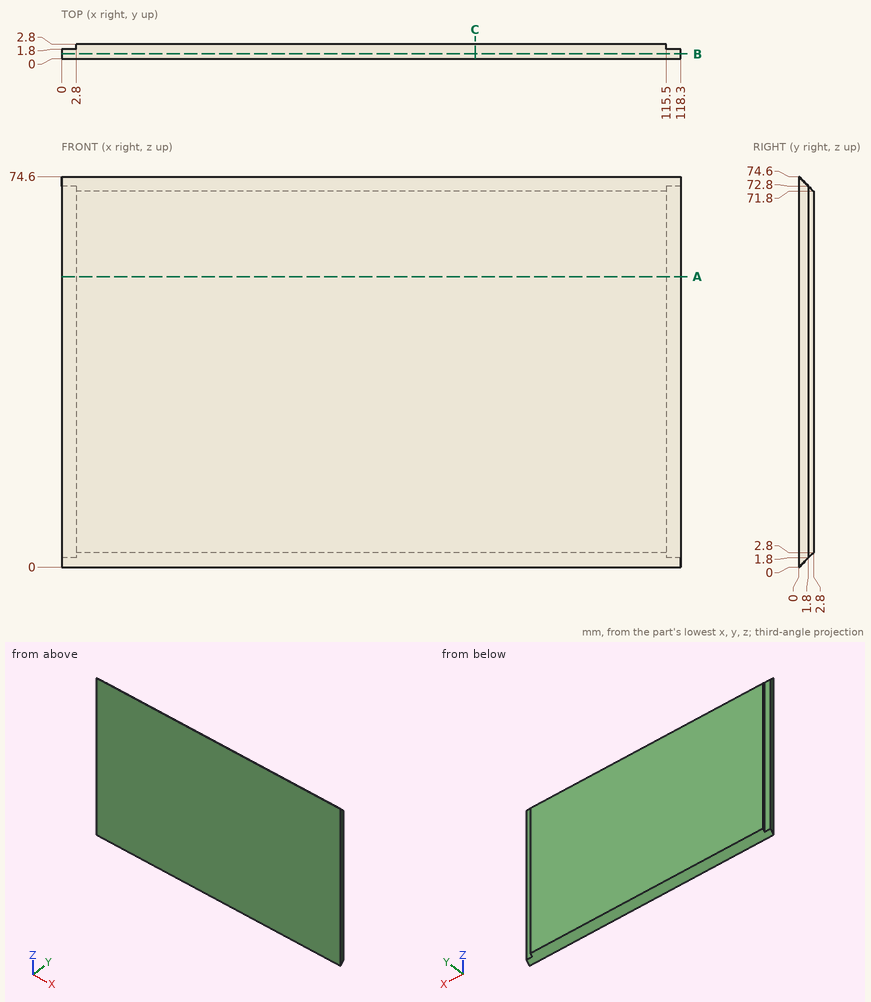
Here's the drawing with two shaded views (mm, measured from the low corner). I have some questions. Round coordinates to 2 decimals unless told otherwise and drop trailing zeros. Write each loop counter-clockwise with the first axis right and the second up, starting at its lowest first coordinate (ties: lowest second). Pieces come first, ordered by that corner, then holes. Notation, with made-up numbers: M -25.5,38.25 L -9.5,38.25 A14 cw -9.5,51.25 Z; hole C 84.25,17 d7. An arc over 180 degrees is marked long. Answer in a Markdown table with one row per item. Add a question column.
Q1. Imagine slicing it at A-A (z = 55.5). Please give me the cut outline in (x, y), then the cut area to 3 significant figures.
Q2. Will these pins go through, and if not, where does the flat tip stop? pin 1 Ø3 at (x, z) = (1, 46.5) entering from +Y; pin 2 Ø1.5 at (x, y) = (56, 1) entering from -Z; pin 3 Ø1.5 at (x, y) = (59.5, 2.5) entering from +Z.
Q3. If I drill on line 1 (X direction, y = 2.2, z = 37); line 2 (Z direction, x = 95.5, y = 0.5); line 3 (Z direction, x = 39.5, y = 1.8), over which ranges is the centre line in solid material (lowest first)? Write a range as from..to.
Q4. Imagine slicing it at B-B (y = 0.9). Please give me the cut outline in (x, z), then the cut area to 3 significant figures.
Q5. Imagine slicing it at C-C (x = 79). Please give me the cut outline in (y, z).
Values:
| question | item | result |
|---|---|---|
| 1 | outline | M 0,0 L 118.3,0 L 118.3,1.8 L 115.5,1.8 L 115.5,2.8 L 2.8,2.8 L 2.8,1.8 L 0,1.8 Z |
| 1 | area | 326 mm^2 |
| 2 | pin 1 | y = 1.8 |
| 2 | pin 2 | z = 0.25 |
| 2 | pin 3 | z = 72.85 |
| 3 | line 1 | 2.8..115.5 |
| 3 | line 2 | 0.5..74.1 |
| 3 | line 3 | 1.8..72.8 |
| 4 | outline | M 0,0.9 L 118.3,0.9 L 118.3,73.7 L 0,73.7 Z |
| 4 | area | 8,610 mm^2 |
| 5 | outline | M 0,0 L 2.8,2.8 L 2.8,71.8 L 0,74.6 Z |
